Geometry check sheet. Reference: the model listing, model coordinates, mm. A direction names the side the tool comes from. Coordinates: 2 decimals unless noted, no trailing zeros. Loops run counter-clockwise (first coordinate to the right, second up) from the corner with the lowest first, then second, coordinate; pieces in that order, holes last.
from build123d import *

# Parameters (mm, degrees)
F1_DEPTH = 25.908
F2_DEPTH = 12.7


with BuildPart() as f1:
    # F0 (on Front) → F1 (new body)
    with BuildSketch(Plane.XZ):
        with BuildLine():
            ThreePointArc((76.078311, 0), (60.586504, 60.586503), (0, 76.078303))
            ThreePointArc((0, 76.078303), (-60.428131, 60.468316), (-75.88172, 0))
            ThreePointArc((-75.88172, 0), (-66.794103, 10.818617), (-54.810586, 18.303441))
            ThreePointArc((-54.810586, 18.303441), (-35.786004, 21.875966), (-17.011248, 17.163621))
            ThreePointArc((-17.011248, 17.163621), (0.091962, 25.558459), (17.225309, 17.225304))
            ThreePointArc((17.225309, 17.225304), (37.337078, 21.900148), (57.435773, 17.169411))
            ThreePointArc((57.435773, 17.169411), (67.981444, 9.91416), (76.078311, 0))
        make_face()
    extrude(amount=F1_DEPTH)

    # F0 (on Front) → F2 (join)
    with BuildSketch(Plane.XZ):
        with BuildLine():
            ThreePointArc((76.078311, 0), (60.586504, 60.586503), (0, 76.078303))
            ThreePointArc((0, 76.078303), (-60.428131, 60.468316), (-75.88172, 0))
            ThreePointArc((-75.88172, 0), (-66.794103, 10.818617), (-54.810586, 18.303441))
            ThreePointArc((-54.810586, 18.303441), (-35.786004, 21.875966), (-17.011248, 17.163621))
            ThreePointArc((-17.011248, 17.163621), (0.091962, 25.558459), (17.225309, 17.225304))
            ThreePointArc((17.225309, 17.225304), (37.337078, 21.900148), (57.435773, 17.169411))
            ThreePointArc((57.435773, 17.169411), (67.981444, 9.91416), (76.078311, 0))
        make_face()
        with BuildLine():
            ThreePointArc((-17.011248, 17.163621), (-35.786004, 21.875966), (-54.810586, 18.303441))
            Line((-54.810586, 18.303441), (-28.897962, -44.034988))
            Line((-28.897962, -44.034988), (0.131057, 3.85879))
            Line((0.131057, 3.85879), (28.504791, -44.034988))
            Line((28.504791, -44.034988), (57.435773, 17.169411))
            ThreePointArc((57.435773, 17.169411), (37.337078, 21.900148), (17.225309, 17.225304))
            ThreePointArc((17.225309, 17.225304), (0.091962, 25.558459), (-17.011248, 17.163621))
        make_face()
        Polygon((0.131057, 3.85879), (-28.897962, -44.034988), (0, -75.88172), (28.504791, -44.034988), align=None)
    extrude(amount=F2_DEPTH)


solid = f1.part
1) Section check D-D on y = -4.25. Record the cut outline in (x, z), and give its area (3 significant figures).
Data:
outline: (-75.88, 0) arc R45.21 cw to (-54.81, 18.3) - (-28.9, -44.03) - (0, -75.88) - (28.5, -44.03) - (57.44, 17.17) arc R45.33 cw to (76.08, 0) arc R61.32 ccw to (0, 76.08) arc R61.32 ccw to start
area: 14,400 mm2
2) Section check A-A on y = -24. Record the cut outline in (x, z), and give its area (3 significant figures).
Data:
outline: (-75.88, 0) arc R45.21 cw to (-54.81, 18.3) arc R45.21 cw to (-17.01, 17.16) arc R21.7 cw to (17.23, 17.23) arc R45.33 cw to (57.44, 17.17) arc R45.33 cw to (76.08, 0) arc R61.32 ccw to (0, 76.08) arc R61.32 ccw to start
area: 7,840 mm2
3) Access from +Z, -Z, +X, -X, +Y, -Y to the whole of each face (thin tool, end or side, straight path). Record for faces 4 (the flat face through (-1, -25.908, 49)), 5 (the flat face through (-42.036, -6.261, -12.429)), 6 (the cylindrical face through (-0.184, -19.212, 25.556)).
Data:
face 4: +Z, -Z, +X, -X, -Y
face 5: -Z, +Y, -Y
face 6: -Z, -Y
4) Material ranges on probe 1 along Y at (x, z) = (-33, 1); probe 2 along Z at (x, y) = (-55, -5.5); probe 3 along X at (y, z) = (-2.25, -16.5), recorded low to high.
Data:
probe 1: y = -12.7 to 0
probe 2: z = 18.22 to 65.3
probe 3: x = -40.34 to 41.52
5) Section check B-B on z = 6.5. Record the cut outline in (x, y).
Data:
outline: (-77.4, -25.91) - (-71.13, -25.91) - (-71.13, 0) - (-77.4, 0) - close; (-49.9, -12.7) - (52.39, -12.7) - (52.39, 0) - (-49.9, 0) - close; (71.32, -25.91) - (77.6, -25.91) - (77.6, 0) - (71.32, 0) - close
6) Section check C-C on x = -13.5. Record the cut outline in (y, z).
Data:
outline: (-25.91, 20.74) - (-12.7, 20.74) - (-12.7, -61) - (0, -61) - (0, 78.38) - (-25.91, 78.38) - close
7) Mould release check, pull along X, two halves, no side actions. Record for faces 1 (the flat face through (14.053, -6.261, -60.181)), 2 (the flat face through (-1, 0, 20)), 3 (the flat face through (1, -12.7, -13)): +X half, -X half, draft (parallel to the pull), parting line (faces both ways), or undercut.
Data:
face 1: +X half
face 2: draft
face 3: undercut
8) Depth check by flat-ended pin: pin 1 (1 mm diameter, centred on y = -13.5, z = 41, fed in from +X); pin 2 (1.5 mm diameter, centred on y = -7, z = 31.5, fed in from -X); pin 3 (2 mm diameter, centred on y = -21, z = -0.5, fed in from +X); pin 4 (3 mm diameter, centred on x = -44.5, z = -14.5, fed in from -Y). Enter the tip coordinate at first touch or a pass-through.
Data:
pin 1: stops at x = 73.96
pin 2: stops at x = -76.81
pin 3: stops at x = 76.22
pin 4: passes through
